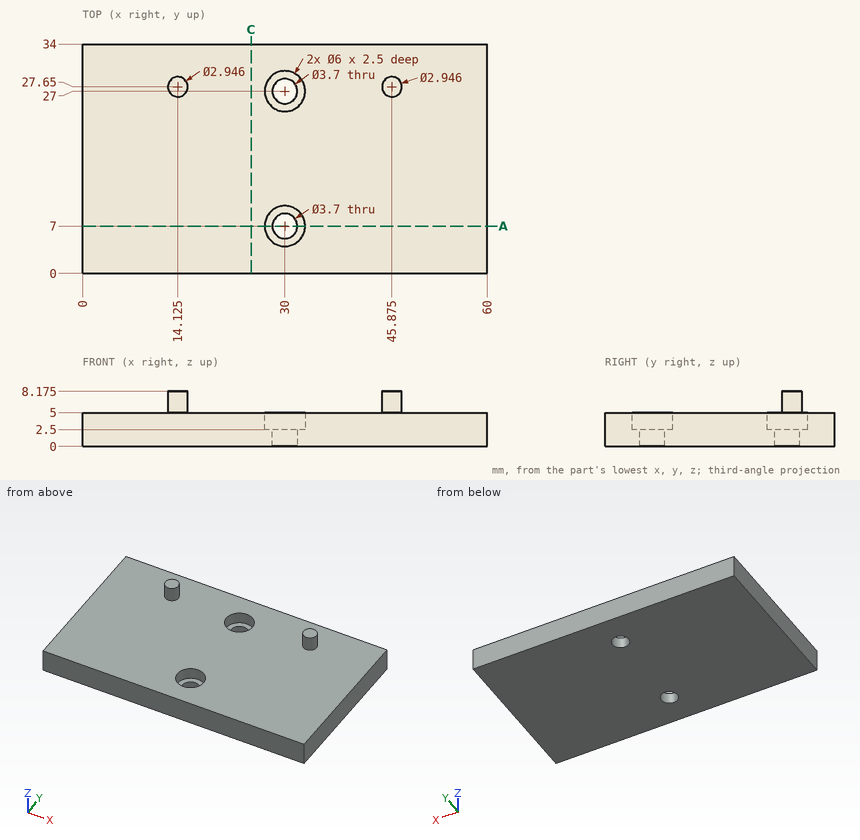
Study the drawing (mm; zero at the part's minimum x, y, z) and answer. Give positions to 0.01 mm unless a question says otherwise; leave off trailing zeros. Write each loop counter-clockwise with the first axis right and the second up, starting at its lowest first coordinate (ties: lowest second). Pieces come first, ordered by that corner, then holes. Notation, with made-up numbers: (57.5, 25.25) -> (109.5, 25.25) arc R13 ccw to (109.5, 33.25) -> close; hole circle Ø5 at (52.25, -21). An arc over 180 degrees is marked (long way). Write item = value, one per line.
Q1. Section C-C on x = 25 is taken. Determine the outline of the cut face in (y, z), and give its area (3 significant figures).
Computed values:
outline = (0, 0) -> (34, 0) -> (34, 5) -> (0, 5) -> close
area = 170 mm^2
Q2. Section A-A on y = 7 is taken. Determine the outline of the cut face in (x, z).
Computed values:
outline = (0, 0) -> (28.15, 0) -> (28.15, 2.5) -> (27, 2.5) -> (27, 5) -> (0, 5) -> close; (31.85, 0) -> (60, 0) -> (60, 5) -> (33, 5) -> (33, 2.5) -> (31.85, 2.5) -> close
Q3. Flat-ended cylindrical pins translate along their axes: pin 1 Ø6.5 at (x, y) = (30, 25.5) entering from +Z; pin 2 Ø4 at (x, z) = (50.5, 2.5) entering from -Y. Find the tip coordinate at first contact, or state that the pin passes through.
Computed values:
pin_1 = 5
pin_2 = 0
Q4. Consider line 1 along Y through (x, z) = (30, 2); line 2 along Y through (x, z) = (30, 3.1); line 3 along Z through (x, y) = (16, 27.5). Determine where each line is inside the solid, lowest interval first.
Computed values:
line_1 = 0 to 5.15, 8.85 to 25.15, 28.85 to 34
line_2 = 0 to 4, 10 to 24, 30 to 34
line_3 = 0 to 5
